Answer from the drawing. Dimensions are ordinates in mm from the lowest x, y and z of the part. A direction names the side the tool comes from. Give positions to 0.01 mm unless a question says otherwise; leave off trailing zeros. Order: outer loops, then holes, each group sorted by start corner. A loop starts at its lowest first (then second) coordinate and runs counter-clockwise, first axis right, second up. Notation, with made-up numbers: (-4.5, -19) - (31.5, -19) arc R8 cw to (31.5, -9) - close; hole circle Ø10 at (-4.75, 9). An arc over 180 degrees is marked (long way). Write each question's results on one line, items separated by ' | '.
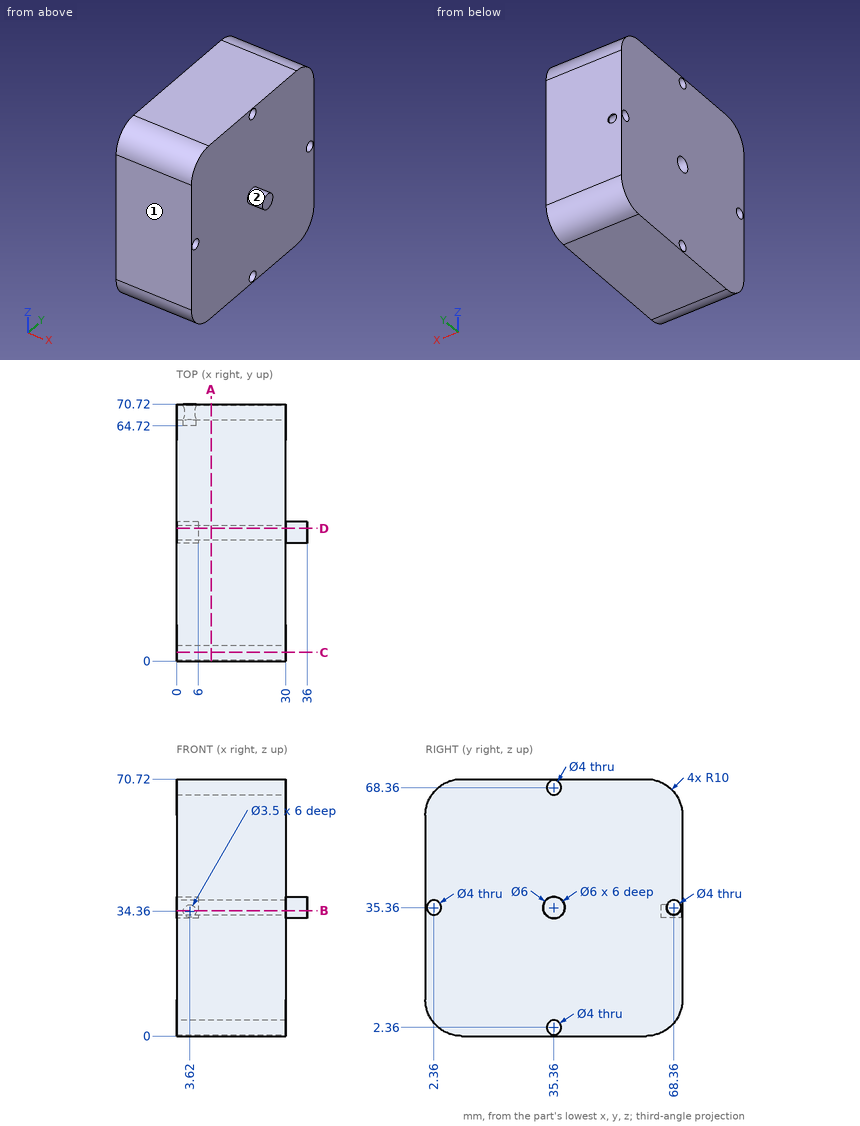
1. Straight lines are drawn through the part: line 1 (Y direction, x = 12.5, z = 35.36); line 2 (Y direction, x = 3.85, z = 35.36); line 3 (Z direction, x = 24, y = 35). For each, find the intervals that lie inside material, in ascending order. Write a range as [from, to].
Answer list:
line 1: [0, 0.36], [4.36, 66.36], [70.36, 70.72] | line 2: [0, 0.36], [4.36, 32.36], [38.36, 64.72] | line 3: [0, 0.39], [4.33, 66.39], [70.33, 70.72]
2. Given P1, Ø3.5, axis at y = 2.36, z = 35.36, coming from the -X side; P2, Ø1, axis at y = 15.5, z = 30, coming from the +X side; P3, Ø1.8, axis at y = 35.5, z = 35, coming from the -X side; P4, Ø1, axis at x = 3, z = 33.5, coming from the +Y side, each flat-ended and moving along its own axis, determine where each tip first touches the part or whether it passes through.
Answer list:
P1: through | P2: x = 30 | P3: x = 6 | P4: y = 64.72
3. A cutting plane is placed at C-C, the plane y = 2.36. Write down the section's boundary in (x, z), then the cut area to 3 significant figures.
Answer list:
outline: (0, 3.55) - (30, 3.55) - (30, 33.36) - (0, 33.36) - close; (0, 37.36) - (30, 37.36) - (30, 67.17) - (0, 67.17) - close | area: 1,790 mm^2
4. A tool of negligible diameter and unlimited length cuts with its end or side. For the marked faces 1 and 2, from which of +Z, -Z, +X, -X, +Y, -Y can it reach the whole face along a straight path? Write none if from no direction.
Answer list:
face 1: +Z, -Z, +X, -X, -Y | face 2: +X
5. A cutting plane is placed at B-B, the plane z = 34.5. Write down the section's boundary in (x, y).
Answer list:
outline: (0, 0) - (30, 0) - (30, 0.55) - (0, 0.55) - close; (0, 4.17) - (30, 4.17) - (30, 32.49) - (36, 32.49) - (36, 38.23) - (30, 38.23) - (30, 66.55) - (5.36, 66.55) - (5.36, 64.72) - (1.88, 64.72) - (1.88, 66.55) - (0, 66.55) - (0, 38.23) - (6, 38.23) - (6, 32.49) - (0, 32.49) - close; (0, 70.17) - (1.88, 70.17) - (1.88, 70.72) - (0, 70.72) - close; (5.36, 70.17) - (30, 70.17) - (30, 70.72) - (5.36, 70.72) - close
6. A cutting plane is placed at D-D, the plane y = 36.5. Write down the section's boundary in (x, z).
Answer list:
outline: (0, 0) - (30, 0) - (30, 0.72) - (0, 0.72) - close; (0, 4) - (30, 4) - (30, 32.59) - (36, 32.59) - (36, 38.13) - (30, 38.13) - (30, 66.72) - (0, 66.72) - (0, 38.13) - (6, 38.13) - (6, 32.59) - (0, 32.59) - close; (0, 70) - (30, 70) - (30, 70.72) - (0, 70.72) - close
7. A cutting plane is placed at A-A, the plane x = 9.5. Write down the section's boundary in (y, z).
Answer list:
outline: (0, 10) arc R10 ccw to (10, 0) - (60.72, 0) arc R10 ccw to (70.72, 10) - (70.72, 60.72) arc R10 ccw to (60.72, 70.72) - (10, 70.72) arc R10 ccw to (0, 60.72) - close; hole circle Ø4 at (2.36, 35.36); hole circle Ø4 at (35.36, 2.36); hole circle Ø4 at (35.36, 68.36); hole circle Ø4 at (68.36, 35.36)
